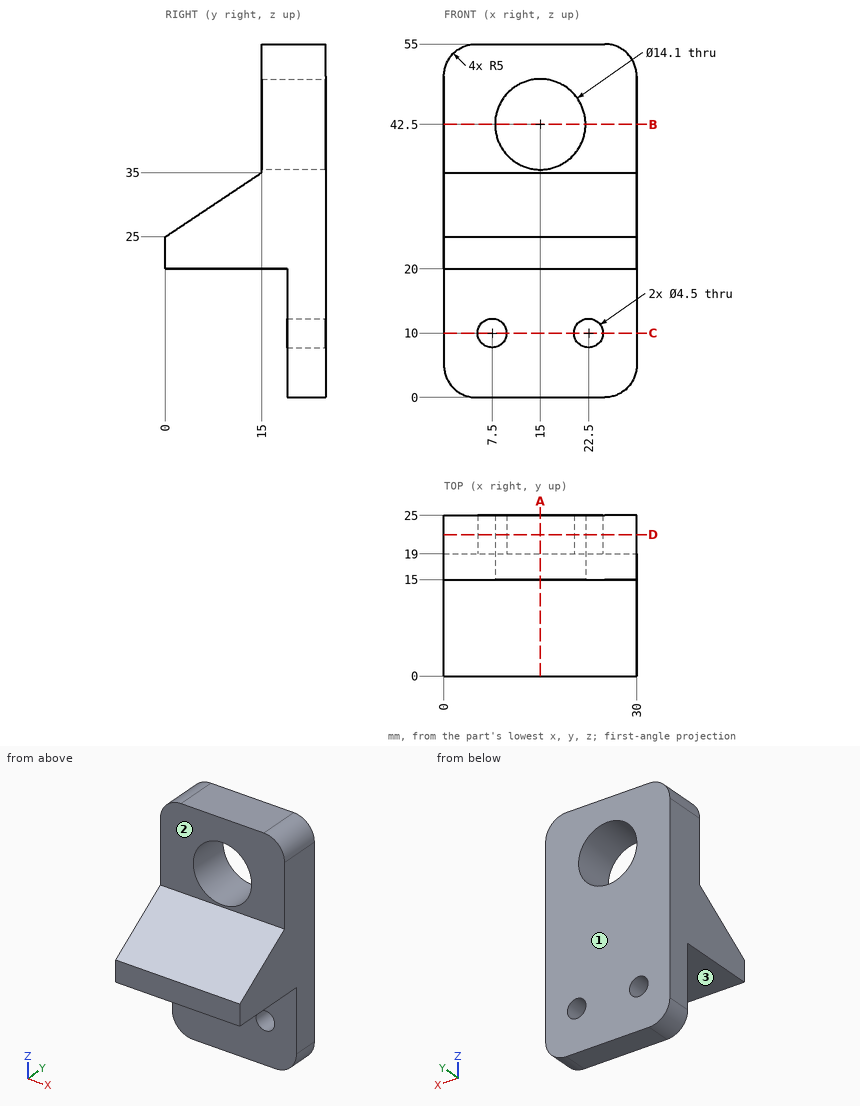
Geometry check sheet. Reference: drawing and pictorial views, mm from the part's lowest x, y, z. A direction names the side the tool comes from. Round coordinates to 2 decimals unless told otherwise and drop trailing zeros. Write each loop counter-clockwise with the first axis right and the second up, starting at its lowest first coordinate (ties: lowest second). Pieces come first, ordered by that corner, then holes.
1. Section check D-D on y = 22. Enter the section's corners in (x, z).
2. Gauge pin test, flat ends, axial feed: P1, Ø1, axis at x = 12, z = 12.5, coming from the -Y side; P2, Ø9.5, axis at x = 13, y = 11, coming from the -Z side; P3, Ø10, axis at x = 13.5, z = 22.5, coming from the -Y side. Record the tip position at first contact, or that the pin passes through.
3. Scan lines: L1, parallel to X at y = 20.8, z = 10; L2, parallel to Z at x = 15, y = 17.75; L3, parallel to Z at x = 15, y = 22.5. Record each from-to range of solid material in increasing order.
4. Section check C-C on z = 10. Enter the section's corners in (x, y).
5. Access from +Z, -Z, +X, -X, +Y, -Y to the whole of each face (thin tool, end or side, straight path). Record for the marked faces 1, 2 and 3.
6. Section check A-A on x = 15. Enter the section's corners in (y, z).
7. Section check B-B on z = 42.5. Enter the section's corners in (x, y), plus the area to 3 significant figures.
Answer:
1. outline: (0, 5) arc R5 ccw to (5, 0) - (25, 0) arc R5 ccw to (30, 5) - (30, 50) arc R5 ccw to (25, 55) - (5, 55) arc R5 ccw to (0, 50) - close; hole circle Ø4.5 at (7.5, 10); hole circle Ø14.1 at (15, 42.5); hole circle Ø4.5 at (22.5, 10)
2. P1: stops at y = 19
2. P2: stops at z = 20
2. P3: stops at y = 0
3. L1: x = 0 to 5.25, 9.75 to 20.25, 24.75 to 30
3. L2: z = 20 to 35.45, 49.55 to 55
3. L3: z = 0 to 35.45, 49.55 to 55
4. outline: (0, 19) - (5.25, 19) - (5.25, 25) - (0, 25) - close; (9.75, 19) - (20.25, 19) - (20.25, 25) - (9.75, 25) - close; (24.75, 19) - (30, 19) - (30, 25) - (24.75, 25) - close
5. face 1: +Z, -Z, +X, -X, +Y
5. face 2: +Z, +X, -X, -Y
5. face 3: -Z, +X, -X, -Y
6. outline: (0, 20) - (19, 20) - (19, 0) - (25, 0) - (25, 35.45) - (15, 35.45) - (15, 35) - (0, 25) - close; (15, 49.55) - (25, 49.55) - (25, 55) - (15, 55) - close
7. outline: (0, 15) - (7.95, 15) - (7.95, 25) - (0, 25) - close; (22.05, 15) - (30, 15) - (30, 25) - (22.05, 25) - close
7. area: 159 mm2
